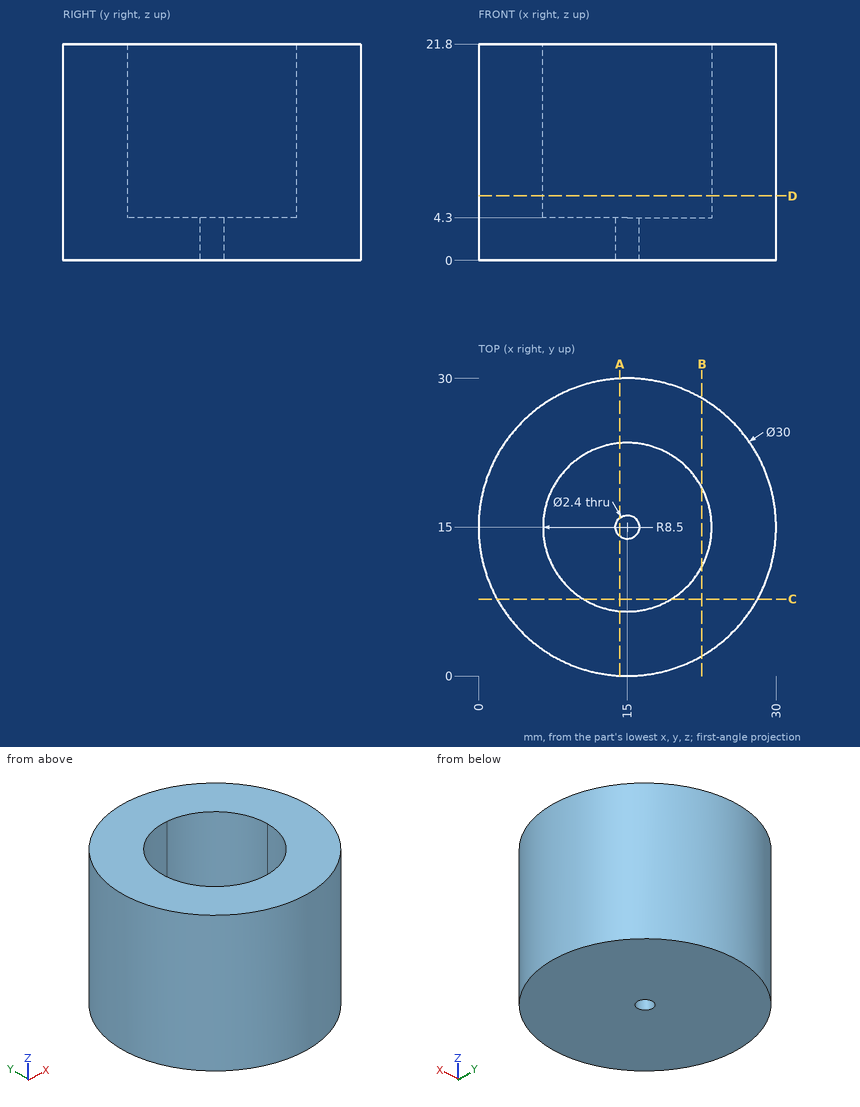
Input: dimensioned drawing with shaded views. Units: mm. Origin: part minimum x, y, z. Coordinates: 2 decimals unless noted, no trailing zeros. Loops run counter-clockwise (first coordinate to the right, second up) from the corner with the lowest first, then second, coordinate; pieces in that order, holes last. Notation, with made-up numbers: M -9.75,77.5 L 45.25,77.5 A19 ccw 45.25,114.5 Z; hole C 41,20.5 d11. An arc over 180 degrees is marked long. One line per item, written item: value. Start each with the question number.
1) Pin query (flat end, axial travel): P1, Ø1, axis at x = 8, z = 16, coming from the -Y side; P2, Ø1.5, axis at x = 5, z = 17.5, coming from the +Y side; P3, Ø5, axis at y = 21, z = 19, coming from the +X side. Return the tip coordinate at first contact, or that it passes through.
2) Cut plane C-C (y = 7.75). Return loops of the section in (x, z), then the cut area to 3 significant figures.
3) Cut plane A-A (x = 14.25). Return loops of the section in (y, z).
4) Cut plane B-B (x = 22.5). Return loops of the section in (y, z), then the cut area to 3 significant figures.
5) Cut plane D-D (z = 6.5). Return loops of the section in (x, y), then the cut area to 3 significant figures.
6) Material intervals for L1, parallel to Y at x = 15, z = 3.35; L2, parallel to Z at x = 11.75, y = 16; L3, parallel to Y at x = 17.25, z = 12.5, sorted ascending. Write a range as from..to.
Evaluation:
1. P1: y = 1.48
1. P2: y = 26.81
1. P3: x = 29.59
2. outline: M 1.87,0 L 28.13,0 L 28.13,21.8 L 19.44,21.8 L 19.44,4.3 L 10.56,4.3 L 10.56,21.8 L 1.87,21.8 Z
2. area: 417 mm^2
3. outline: M 0.02,0 L 14.06,0 L 14.06,4.3 L 6.53,4.3 L 6.53,21.8 L 0.02,21.8 Z; M 15.94,0 L 29.98,0 L 29.98,21.8 L 23.47,21.8 L 23.47,4.3 L 15.94,4.3 Z
4. outline: M 2.01,0 L 27.99,0 L 27.99,21.8 L 19,21.8 L 19,4.3 L 11,4.3 L 11,21.8 L 2.01,21.8 Z
4. area: 426 mm^2
5. outline: C 15,15 d30; hole M 15,6.5 A8.5 ccw 23.5,15 A8.5 ccw 15,23.5 A8.5 ccw Z
5. area: 480 mm^2
6. L1: 0..13.8, 16.2..30
6. L2: 0..4.3
6. L3: 0.17..6.8, 23.2..29.83
